Work out the finished part from the listing and answer in its coordinate system (mm). A direction names the side the tool comes from. Give positions to 0.01 mm unless a question says otherwise; leave off trailing zeros. Loops run counter-clockwise (first coordinate to the right, second up) from the corner with the lowest first, then second, coordinate; pieces in that order, holes last.
```python
from build123d import *

# Parameters (mm, degrees)
ESQUISSE15_W             = 106
ESQUISSE15_H             = 176
ESQUISSE15_W_2           = 100
ESQUISSE15_H_2           = 170
BOSS_EXTRU_9_DEPTH       = 70
CONG_1_R                 = 3
ESQUISSE18_W             = 106
ESQUISSE18_H             = 176
BOSS_EXTRU_10_DEPTH      = 3
CONG_2_R                 = 3
ESQUISSE22_R             = 10.869506495
ENL_V_MAT_EXTRU_5_DEPTH  = 3
ESQUISSE23_W             = 14
ESQUISSE23_H             = 38
ENL_V_MAT_EXTRU_6_DEPTH  = 3
ESQUISSE24_W             = 3
ESQUISSE24_H             = 20
ENL_V_MAT_EXTRU_7_DEPTH  = 3
ESQUISSE26_R             = 2.5
ENL_V_MAT_EXTRU_11_DEPTH = 3
ESQUISSE28_W             = 13
ESQUISSE28_H             = 9
ENL_V_MAT_EXTRU_13_DEPTH = 3
D_GAGEMENT_03_D          = 10.9248
ESQUISSE43_W             = 10
ESQUISSE43_H             = 5
BOSS_EXTRU_11_DEPTH      = 3
ESQUISSE44_W             = 3
ESQUISSE44_H             = 9
BOSS_EXTRU_12_DEPTH      = 3


with BuildPart() as part:
    # Esquisse15 → Boss.-Extru.9 (new body)
    with BuildSketch(Plane(origin=(0, 0, 0), x_dir=(1, 0, 0), z_dir=(0, 1, 0))):
        Rectangle(ESQUISSE15_W, ESQUISSE15_H)
        Rectangle(ESQUISSE15_W_2, ESQUISSE15_H_2, mode=Mode.SUBTRACT)
    extrude(amount=BOSS_EXTRU_9_DEPTH)

    # Congé1
    cong_1_edges = [part.edges().sort_by_distance(p)[0] for p in [
        (-53, 35, -88),
        (53, 35, -88),
        (53, 35, 88),
        (-53, 35, 88),
    ]]
    fillet(cong_1_edges, radius=CONG_1_R)

    # Esquisse18 → Boss.-Extru.10 (add)
    with BuildSketch(Plane.XZ):
        Rectangle(ESQUISSE18_W, ESQUISSE18_H)
    extrude(amount=BOSS_EXTRU_10_DEPTH)

    # Congé2
    cong_2_edges = [part.edges().sort_by_distance(p)[0] for p in [
        (53, -1.5, 88),
        (53, -1.5, -88),
        (-53, -1.5, -88),
        (-53, -1.5, 88),
    ]]
    fillet(cong_2_edges, radius=CONG_2_R)

    # Esquisse22 → Enlèv. mat.-Extru.5 (cut)
    with BuildSketch(Plane(origin=(0, 0, 0), x_dir=(1, 0, 0), z_dir=(0, 1, 0))):
        with Locations((0, -60)):
            Circle(ESQUISSE22_R)
    extrude(amount=-ENL_V_MAT_EXTRU_5_DEPTH, mode=Mode.SUBTRACT)

    # Esquisse23 → Enlèv. mat.-Extru.6 (cut)
    with BuildSketch(Plane(origin=(0, 0, 0), x_dir=(1, 0, 0), z_dir=(0, 1, 0))):
        with Locations((30.434753248, -60)):
            Rectangle(ESQUISSE23_W, ESQUISSE23_H)
    extrude(amount=-ENL_V_MAT_EXTRU_6_DEPTH, mode=Mode.SUBTRACT)

    # Esquisse24 → Enlèv. mat.-Extru.7 (cut)
    with BuildSketch(Plane(origin=(0, 0, 0), x_dir=(1, 0, 0), z_dir=(0, 1, 0))):
        with Locations((-30.434753248, -60)):
            Rectangle(ESQUISSE24_W, ESQUISSE24_H)
    extrude(amount=-ENL_V_MAT_EXTRU_7_DEPTH, mode=Mode.SUBTRACT)

    # Esquisse26 → Enlèv. mat.-Extru.11 (cut)
    with BuildSketch(Plane(origin=(0, 0, 85), x_dir=(-1, 0, 0), z_dir=(0, 0, -1))):
        with Locations((-25, 52.5)):
            Circle(ESQUISSE26_R)
        with Locations((25, 52.5)):
            Circle(ESQUISSE26_R)
    extrude(amount=-ENL_V_MAT_EXTRU_11_DEPTH, mode=Mode.SUBTRACT)

    # Esquisse28 → Enlèv. mat.-Extru.13 (cut)
    with BuildSketch(Plane(origin=(0, 0, 85), x_dir=(-1, 0, 0), z_dir=(0, 0, -1))):
        with Locations((0, 52.5)):
            Rectangle(ESQUISSE28_W, ESQUISSE28_H)
    extrude(amount=-ENL_V_MAT_EXTRU_13_DEPTH, mode=Mode.SUBTRACT)

    # Dégagement #03 (through all)
    with Locations(Plane(origin=(-50, 70, 23.760275735), x_dir=(1, 0, 0), z_dir=(0, 0.573576436, 0.819152044))):
        with Locations((10.736336361, -22.988358748)):
            Hole(D_GAGEMENT_03_D / 2)

    # Esquisse43 → Boss.-Extru.11 (add)
    with BuildSketch(Plane.XY.offset(88)):
        with Locations((-1.5, 54.5)):
            Rectangle(ESQUISSE43_W, ESQUISSE43_H)
    extrude(amount=-BOSS_EXTRU_11_DEPTH)

    # Esquisse44 → Boss.-Extru.12 (add)
    with BuildSketch(Plane.XY.offset(88)):
        with Locations((5, 52.5)):
            Rectangle(ESQUISSE44_W, ESQUISSE44_H)
    extrude(amount=-BOSS_EXTRU_12_DEPTH)


solid = part.part
```
Q1. Section A-A on x = 0 is taken. Give the vertices of the cut face in (y, z).
Q2. Section B-B on z = 60 is taken. Give the vertices of the cut face in (x, y).
Q3. Given pin 1 (17.5 mm diameter, centred on x = 0, z = 60, fed in from -Y); pin 2 (8 mm diameter, centred on x = 38, z = 8.5, fed in from +Y), each flat-ended and moving along its own axis, determine where each tip first touches the part or whether it passes through.
Q4. Section D-D on y = 31.5 is taken. Give the vertices of the cut face in (x, z).
Q5. Determine the mould class of faces 4 (the face through (-1, 34, 88)), 5 (the face through (-1, 34, -88)), 6 (the face through (27, 54, 86)), 7 (the face through (-50, 35, 1)) for opening direction Z: +Z half, -Z half, draft (parallel to the pull), parting line (faces both ways), or undercut.
Q6. Which of the six approach directions +Z, -Z, +X, -X, +Y, -Y give full straight-line access (tool end or side, diameter ignored) to faces 1 (the face through (-23, 54, 86)), 2 (the face through (53, 34, -1)), 3 (the face through (-1, 35, 85))?
Q7. Consider line 1 along Z through (x, y) = (-1, 3); line 2 along X through (y, z) = (40.5, 68); line 3 along Y through (x, z) = (25, 86.45). Determine where each line is inside the solid, lowest interval first.
Q8. Section C-C on x = -25 is taken. Give the vertices of the cut face in (y, z), plus the area to 3 significant figures.
Check result:
1. outline: (-3, -88) - (70, -88) - (70, -85) - (0, -85) - (0, 49.13) - (-3, 49.13) - close; (-3, 70.87) - (0, 70.87) - (0, 85) - (48, 85) - (48, 88) - (-3, 88) - close; (52, 85) - (70, 85) - (70, 88) - (52, 88) - close
2. outline: (-53, -3) - (-31.93, -3) - (-31.93, 0) - (-50, 0) - (-50, 70) - (-53, 70) - close; (-28.93, -3) - (-10.87, -3) - (-10.87, 0) - (-28.93, 0) - close; (10.87, -3) - (23.43, -3) - (23.43, 0) - (10.87, 0) - close; (37.43, -3) - (53, -3) - (53, 70) - (50, 70) - (50, 0) - (37.43, 0) - close
3. pin 1: passes through
3. pin 2: stops at y = 0
4. outline: (-53, -85) arc R3 ccw to (-50, -88) - (50, -88) arc R3 ccw to (53, -85) - (53, 85) arc R3 ccw to (50, 88) - (-50, 88) arc R3 ccw to (-53, 85) - close; hole (-50, -85) - (50, -85) - (50, 85) - (-50, 85) - close
5. face 4: +Z half
5. face 5: -Z half
5. face 6: draft
5. face 7: undercut
6. face 1: +Z
6. face 2: +Z, -Z, +X, +Y, -Y
6. face 3: +Y
7. line 1: z = -88 to -85, 85 to 88
7. line 2: x = -53 to -50, 50 to 53
7. line 3: y = -3 to 50, 55 to 70
8. outline: (-3, -88) - (70, -88) - (70, -85) - (0, -85) - (0, 85) - (50, 85) - (50, 88) - (-3, 88) - close; (55, 85) - (70, 85) - (70, 88) - (55, 88) - close
8. area: 933 mm2
